Answer from the drawing. Dimensions are ordinates in mm from the lowest x, y and z of the part. A direction names the side the tool comes from. Round coordinates to 2 decimals unless told otherwise and drop trailing zeros. Write each loop counter-clockwise with the first axis right and the second up, starting at its lowest first coordinate (ties: lowest second). Pieces come first, ordered by that corner, then holes. Notation, with made-up numbers: (-7.5, 54) -> (47.5, 54) arc R5 ccw to (47.5, 58) -> close; hole circle Ø4 at (-37.5, -0.75). An arc over 180 degrees is marked (long way). Return JSON: item names as keys, results as strings. Group by question number.
(1) A cutting plane is placed at C-C on x = 16. Give the vertices of the cut face in (y, z) (1 decimal).
(2) The mould has two halves that part along X. Classify the marked faces 1, 2, 3 and 4: released by +X, released by -X, zero draft, split by the parting line, or undercut.
(3) A cutting plane is placed at A-A on y = 24.5. Give the vertices of the cut face in (x, z) (1 decimal), then the cut area to 3 significant figures.
(4) Straight lines are drawn through the part: line 1 (Z direction, x = 121.2, y = 99.8) (1 decimal); line 2 (Y direction, x = 85.5, z = 35.5) (1 decimal); line 3 (X direction, y = 64, z = 37.5) (1 decimal). For each, find the intervals that lie inside material, in ascending order.
(5) For the marked faces 5 and 6, determine the directions among +Z, -Z, +X, -X, +Y, -Y from which every point of the face is accessible in a straight line to the end or side of a thin tool.
(6) A cutting plane is placed at B-B on x = 121.2. Give the vertices of the cut face in (y, z) (1 decimal), then the cut area to 3 significant figures.
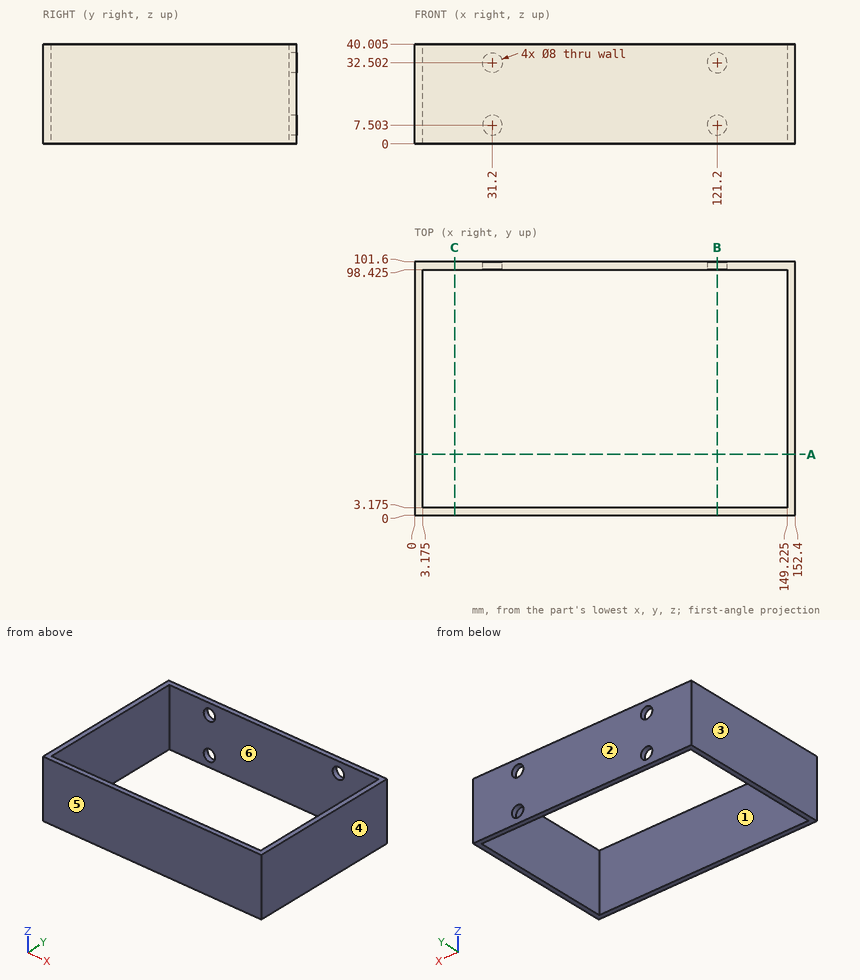
Checks:
{
 "1": {"outline": "(0, 0) -> (3.2, 0) -> (3.2, 40) -> (0, 40) -> close; (98.4, 0) -> (101.6, 0) -> (101.6, 40) -> (98.4, 40) -> close"},
 "2": {"face 1": "undercut", "face 2": "zero draft", "face 3": "released by -X", "face 4": "released by +X"},
 "3": {"outline": "(0, 0) -> (3.2, 0) -> (3.2, 40) -> (0, 40) -> close; (149.2, 0) -> (152.4, 0) -> (152.4, 40) -> (149.2, 40) -> close", "area": "254 mm^2"},
 "4": {"line 1": "z = 0 to 3.5, 11.5 to 28.5, 36.5 to 40", "line 2": "y = 0 to 3.2, 98.4 to 101.6", "line 3": "x = 0 to 3.2, 149.2 to 152.4"},
 "5": {"face 5": "+Z, -Z, +X, -X, -Y", "face 6": "+Z, -Z"},
 "6": {"outline": "(0, 0) -> (3.2, 0) -> (3.2, 40) -> (0, 40) -> close; (98.4, 0) -> (101.6, 0) -> (101.6, 3.5) -> (98.4, 3.5) -> close; (98.4, 11.5) -> (101.6, 11.5) -> (101.6, 28.5) -> (98.4, 28.5) -> close; (98.4, 36.5) -> (101.6, 36.5) -> (101.6, 40) -> (98.4, 40) -> close", "area": "203 mm^2"}
}
